Input: part model. Units: mm. Frame: model coordinates. Face numbers are marked on the shaded views. A direction names the side the tool comes from. Give positions to 0.01 mm unless a question says otherwise; leave off trailing zeros. Loops run counter-clockwise (first coordinate to the right, second up) from the corner with the lowest first, then second, coordinate; pieces in that order, holes last. Notation, with made-up numbers: (-16.5, 12) -> (13.5, 12) arc R14 ccw to (13.5, 35) -> close; hole circle Ø8 at (65.25, 17.25). An arc over 180 degrees is marked (long way). One line per question, with ' | ' between items.
from build123d import *

# Parameters (mm, degrees)
EXTRUDE_7_DEPTH     = 6.4
EXTRUDE_8_DEPTH     = 1
FILLET_1_R          = 2
FILLET_4_R          = 3
CUT_EXTRUDE_1_DEPTH = 36.117222337


with BuildPart() as part:
    # 草图1 → 凸台-拉伸7 (new body)
    with BuildSketch(Plane(origin=(0, 0, 0), x_dir=(1, 0, 0), z_dir=(0, 1, 0))):
        with BuildLine():
            ThreePointArc((-8.25, 6.915846718), (0, 7.441530126), (8.25, 6.915846718))
            ThreePointArc((8.25, 6.915846718), (2.55299652, 23.258172204), (-9.25, 35.915846718))
            ThreePointArc((-9.25, 35.915846718), (-6.599997803, 21.489984725), (-8.25, 6.915846718))
        make_face()
        with BuildLine():
            ThreePointArc((-5.663467174, 30.373218023), (-4.570302184, 19.788295497), (-5.654744598, 9.202475772))
            ThreePointArc((-5.654744598, 9.202475772), (0.10266918, 9.441451462), (5.859323518, 9.184831872))
            ThreePointArc((5.859323518, 9.184831872), (1.732970319, 20.668203024), (-5.663467174, 30.373218023))
        make_face(mode=Mode.SUBTRACT)
    extrude(amount=EXTRUDE_7_DEPTH)

    # 草图1<9> → 凸台-拉伸8 (add)
    with BuildSketch(Plane(origin=(0, 0, 0), x_dir=(1, 0, 0), z_dir=(0, 1, 0))):
        with BuildLine():
            ThreePointArc((-11.257417673, 38.414736689), (-7.630939872, 22.203928266), (-9.628954872, 5.713034203))
            ThreePointArc((-9.628954872, 5.713034203), (-0.121629419, 6.44141455), (9.388395867, 5.749175976))
            ThreePointArc((9.388395867, 5.749175976), (2.941633426, 24.53181947), (-11.257417673, 38.414736689))
        make_face()
    extrude(amount=-EXTRUDE_8_DEPTH)

    # 圆角1
    fillet_1_edges = [part.edges().sort_by_distance(p)[0] for p in [
        (-8.25, 3.2, -6.915846718),
        (-9.25, 3.2, -35.915846718),
        (8.25, 3.2, -6.915846718),
    ]]
    fillet(fillet_1_edges, radius=FILLET_1_R)

    # 圆角4
    fillet_4_edges = [part.edges().sort_by_distance(p)[0] for p in [
        (9.388395867, -0.5, -5.749175976),
        (-9.628954872, -0.5, -5.713034203),
        (-11.257417673, -0.5, -38.414736689),
    ]]
    fillet(fillet_4_edges, radius=FILLET_4_R)

    # 草图1<10> → 切除-拉伸1 (cut, through all)
    with BuildSketch(Plane(origin=(0, 0, 0), x_dir=(1, 0, 0), z_dir=(0, 1, 0))):
        with BuildLine():
            ThreePointArc((-5.654744598, 9.202475772), (0.10266918, 9.441451462), (5.859323518, 9.184831872))
            ThreePointArc((5.859323518, 9.184831872), (1.732970319, 20.668203024), (-5.663467174, 30.373218023))
            ThreePointArc((-5.663467174, 30.373218023), (-4.570302184, 19.788295497), (-5.654744598, 9.202475772))
        make_face()
    extrude(amount=-CUT_EXTRUDE_1_DEPTH, mode=Mode.SUBTRACT)


solid = part.part
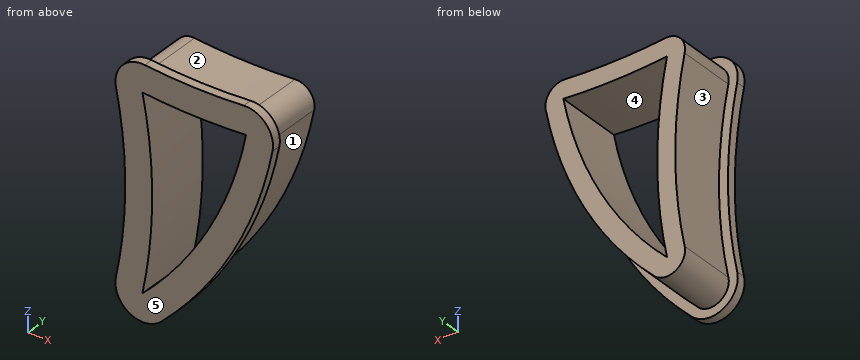
1. Reachability of the marked faces 4 and 5 from +Z, -Z, +X, -X, +Y, -Y: full face, straight path, thin tool, end or side. Return the list, or none.
Determined:
face 4: +Y, -Y | face 5: +Z, -Z, +X, -X, -Y
2. Section query B-B (z = -28.5). Output: boundary loops of the cut face in (x, y).
Determined:
outline: (-8.35, -1) -> (-5.31, -1) -> (-5.31, 6.4) -> (-7.34, 6.4) -> (-7.34, 0) -> (-8.35, 0) -> close; (-3.84, -1) -> (0.11, -1) -> (0.11, 0) -> (-1.19, 0) -> (-1.19, 6.4) -> (-3.84, 6.4) -> close
3. Pull-direction query (X, two-part tool) for the marked faces 1, 2 and 3; classes: pulls with the +X half, pulls with the -X half, needs draft (parallel to the pull), parting line crosses it, or undercut.
Determined:
face 1: pulls with the +X half | face 2: undercut | face 3: pulls with the -X half
4. Ray query, line 1 along Y through (x, z) = (-0.25, -28.5); line 2 along X through (y, z) = (4, -25); line 3 along X through (y, z) = (2.25, -28.75). Return the intervals inside material, ascending. Write a range as from..to.
Determined:
line 1: y = -1..0 | line 2: x = -6.84..-4.83, -1..1.44 | line 3: x = -7.38..-5.35, -4.07..-1.4
5. Pin query (flat end, axial travel): P1, Ø1, axis at x = -4, y = 2, coming from the +Z side; P2, Ø4, axis at y = 1.5, z = -28.5, coming from the +X side; P3, Ø1.5, axis at x = 1, y = 0.5, coming from the -Z side. Return the tip coordinate at first contact, or that it passes through.
Determined:
P1: stops at z = -7.29 | P2: stops at x = 1.13 | P3: stops at z = -28.08
6. Section query A-A (x = -0.25). Output: boundary loops of the cut face in (y, z).
Determined:
outline: (-1, -28.94) -> (0, -28.94) -> (0, -27.34) -> (6.4, -27.34) -> (6.4, -23.93) -> (-1, -23.93) -> close; (-1, -9.44) -> (6.4, -9.44) -> (6.4, -7.44) -> (0, -7.44) -> (0, -6.44) -> (-1, -6.44) -> close
